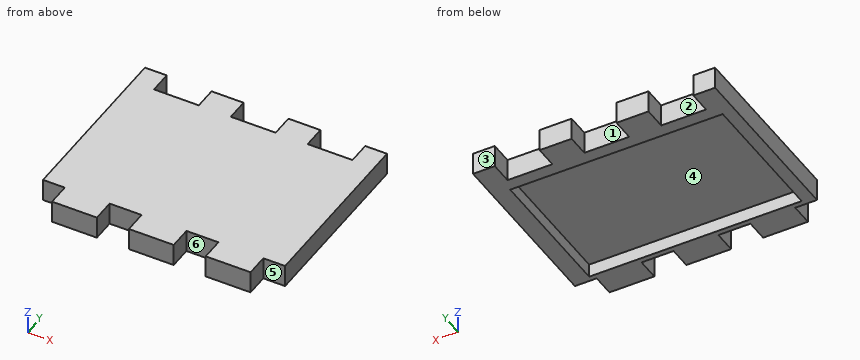
Autodesk Inventor part; units mm, degrees
ref_plane "YZ Plane" through (0, 0, 0) normal (1, 0, 0) x (0, 1, 0)
ref_plane "XZ Plane" through (0, 0, 0) normal (0, 1, 0) x (-1, 0, 0)
ref_plane "XY Plane" through (0, 0, 0) normal (0, 0, 1) x (1, 0, 0)
sketch "Sketch1" plane through (0, 0, 0) normal (0, 0, 1) x (1, 0, 0)
  line L0 (68.58, 6.35) -> (68.58, 57.15)
  line L1 (68.58, 57.15) -> (0, 57.15)
  line L2 (0, 57.15) -> (0, 6.35)
  line L3 (40.64, 6.35) -> (40.64, 0)
  line L4 (27.94, 6.35) -> (27.94, 0)
  line L5 (27.94, 0) -> (40.64, 0)
  line L6 (27.94, 6.35) -> (18.8722, 6.35)
  line L7 (18.8722, 6.35) -> (18.8722, 0)
  line L8 (18.8722, 0) -> (6.1722, 0)
  line L9 (6.1722, 0) -> (6.1722, 6.35)
  line L10 (40.64, 6.35) -> (49.7078, 6.35)
  line L11 (49.7078, 6.35) -> (49.7078, 0)
  line L12 (49.7078, 0) -> (62.4078, 0)
  line L13 (62.4078, 0) -> (62.4078, 6.35)
  line L14 (6.1722, 0) -> (18.8722, 0)
  line L15 (27.94, 0) -> (40.64, 0)
  line L16 (49.7078, 0) -> (62.4078, 0)
  line L17 (27.94, 6.35) -> (18.8722, 6.35)
  line L18 (6.1722, 6.35) -> (0, 6.35)
  line L19 (40.64, 6.35) -> (49.7078, 6.35)
  line L20 (62.4078, 6.35) -> (68.58, 6.35)
  point P0 (0, 0)
  dimension "d0" = 68.58
  dimension "d1" = 50.8
extrude "Extrusion1" add sketch "Sketch1" against normal blind 6.35
sketch "Sketch2" plane through (0, 0, 0) normal (0, 0, 1) x (1, 0, 0)
  line L0 (0, 6.35) -> (6.1722, 6.35)
  line L1 (6.1722, 50.8) -> (6.1722, 57.15)
  line L2 (0, 57.15) -> (68.58, 57.15)
  line L3 (49.7078, 6.35) -> (40.64, 6.35)
  line L4 (40.64, 50.8) -> (40.64, 57.15)
  line L5 (18.8722, 0) -> (18.8722, 6.35)
  line L6 (18.8722, 50.8) -> (18.8722, 57.15)
  line L7 (27.94, 0) -> (27.94, 6.35)
  line L8 (27.94, 50.8) -> (27.94, 57.15)
  line L9 (49.7078, 50.8) -> (49.7078, 57.15)
  line L10 (68.58, 6.35) -> (62.4078, 6.35)
  line L11 (62.4078, 50.8) -> (62.4078, 57.15)
  line L12 (0, 57.15) -> (0, 50.8)
  line L13 (68.58, 57.15) -> (68.58, 6.35)
  line L14 (49.7078, 50.8) -> (62.4078, 50.8)
  line L15 (6.1722, 50.8) -> (18.8722, 50.8)
  line L16 (27.94, 50.8) -> (40.64, 50.8)
  line L17 (27.94, 57.15) -> (40.64, 57.15)
  point P0 (0, 0)
extrude "Extrusion2" cut sketch "Sketch2" against normal blind 6.35
sketch "Sketch3" plane through (0, 0, -6.35) normal (0, 0, -1) x (-1, 0, 0)
  line L0 (-63.699, 7.8373) -> (-3.501, 7.8373)
  line L1 (-3.501, 7.8373) -> (-3.501, 47.2073)
  line L2 (-3.501, 47.2073) -> (-63.699, 47.2073)
  line L3 (-63.699, 47.2073) -> (-63.699, 7.8373)
  point P0 (0, 0)
  dimension "d15" = 60.198
  dimension "d16" = 39.37
extrude "Extrusion3" cut sketch "Sketch3" against normal blind 3.81
properties part number "front-flat"
Build history of the part. All positions in model axes, mm. Face numbers are marked on the shaded views. A direction names the side the tool comes from. Coordinates: 2 decimals unless noted, no trailing zeros. Write each loop counter-clockwise with the first axis right and the second up, starting at its lowest first coordinate (ties: lowest second). Pieces come first, ordered by that corner, then holes. Notation, with made-up numbers: (-29, 74.5) -> (2, 74.5) arc R26 ccw to (2, 96.5) -> close; hole circle Ø5 at (26, -38). An arc over 180 degrees is marked (long way). Use CSV: the item, a comma, the result in double quotes. Start each with the question number.
Q1. Pull direction X, two halves, no side cores. Call the marked faces 1, 2 and 3: released by +X, released by -X, zero draft, split by the parting line, or undercut.
Q2. Cut at B-B, the plane y = 16. List the corners of the cut face in (x, z).
Q3. Drill centre lines: probe 1 along X at (y, z) = (4, -1.5); probe 2 along Y at (x, z) = (6.5, -5.5); probe 3 along X at (y, z) = (45.5, -5.5). Where is each one in solid material? Low to high.
Q4. Cut at D-D, the plane x = 12. List the corners of the cut face in (y, z).
Q5. 3-axis set-ups, long thin cutter, end or side, ignore diameter. For the marked faces 4, 5 and 6: which of +Z, -Z, +X, -X, +Y, -Y reach the whole face in a straight line?
Q6. Flat gauge pins, fed straight in: pin 1 Ø1.5 at (x, y) = (61, 42.5) entering from +Z; pin 2 Ø1.9 at (y, z) = (2.5, -2) entering from +X; pin 3 Ø1 at (x, z) = (16.5, -3) entering from +Y; pin 4 Ø1.9 at (x, z) = (46, -1.5) entering from -Y. Where does each tip first touch, or does it go through?
Q7. Cut at C-C, the plane z = -1. List the corners of the cut face in (x, y).
Checked values:
1,face 1,"undercut"
1,face 2,"undercut"
1,face 3,"zero draft"
2,outline,"(0, -6.35) -> (3.5, -6.35) -> (3.5, -2.54) -> (63.7, -2.54) -> (63.7, -6.35) -> (68.58, -6.35) -> (68.58, 0) -> (0, 0) -> close"
3,probe 1,"x = 6.17 to 18.87, 27.94 to 40.64, 49.71 to 62.41"
3,probe 2,"y = 0 to 7.84, 47.21 to 50.8"
3,probe 3,"x = 0 to 3.5, 63.7 to 68.58"
4,outline,"(0, -6.35) -> (7.84, -6.35) -> (7.84, -2.54) -> (47.21, -2.54) -> (47.21, -6.35) -> (50.8, -6.35) -> (50.8, 0) -> (0, 0) -> close"
5,face 4,"-Z"
5,face 5,"+Z, -Z, +X, -Y"
5,face 6,"+Z, -Z, -Y"
6,pin 1,"stops at z = 0"
6,pin 2,"stops at x = 62.41"
6,pin 3,"stops at y = 50.8"
6,pin 4,"stops at y = 6.35"
7,outline,"(0, 6.35) -> (6.17, 6.35) -> (6.17, 0) -> (18.87, 0) -> (18.87, 6.35) -> (27.94, 6.35) -> (27.94, 0) -> (40.64, 0) -> (40.64, 6.35) -> (49.71, 6.35) -> (49.71, 0) -> (62.41, 0) -> (62.41, 6.35) -> (68.58, 6.35) -> (68.58, 57.15) -> (62.41, 57.15) -> (62.41, 50.8) -> (49.71, 50.8) -> (49.71, 57.15) -> (40.64, 57.15) -> (40.64, 50.8) -> (27.94, 50.8) -> (27.94, 57.15) -> (18.87, 57.15) -> (18.87, 50.8) -> (6.17, 50.8) -> (6.17, 57.15) -> (0, 57.15) -> close"
